```python
from build123d import *

# Parameters (mm, degrees)
BOSS_EXTRUDE1_DEPTH     = 3.175
CUT_EXTRUDE1_DEPTH      = 95.24196383
CUT_EXTRUDE1_DEPTH_BACK = 95.24196383
SKETCH3_W               = 12.7
SKETCH3_H               = 3.175


with BuildPart() as part:
    # Sketch2 → Boss-Extrude1 (new body)
    with BuildSketch(Plane.XY):
        Polygon((13.027299887, 62.53449296), (12.7, 62.861792847), (0, 62.861792847), (0, 0), (70.141728817, 0), (70.141728817, 5.42006403), (67.896664787, 3.175), (58.916408666, 12.155256121), (61.161472696, 14.400320151), (52.181216575, 23.380576272), (49.936152545, 21.135512242), (40.955896424, 30.115768363), (43.200960454, 32.360832393), (34.220704333, 41.341088515), (31.975640303, 39.096024484), (22.995384182, 48.076280605), (25.240448212, 50.321344636), (16.260192091, 59.301600757), (14.015128061, 57.056536726), (10.782235857, 60.28942893), align=None)
    extrude(amount=BOSS_EXTRUDE1_DEPTH)

    # Sketch3 → Cut-Extrude1 (cut, two sides: drawn at the far end of the back side and taken through both)
    with BuildSketch(Plane.XY.offset(3.175).offset(-CUT_EXTRUDE1_DEPTH_BACK)):
        with Locations((44.741728817, 1.5875)):
            Rectangle(SKETCH3_W, SKETCH3_H)
        with Locations((19.341728817, 1.5875)):
            Rectangle(SKETCH3_W, SKETCH3_H)
    extrude(amount=CUT_EXTRUDE1_DEPTH + CUT_EXTRUDE1_DEPTH_BACK, mode=Mode.SUBTRACT)


solid = part.part
```
Work out the finished part from the listing and answer in its coordinate system (mm). A direction names the side the tool comes from. Give positions to 0.01 mm unless a question says otherwise; leave off trailing zeros. Order: outer loops, then holes, each group sorted by start corner. A loop starts at its lowest first (then second) coordinate and runs counter-clockwise, first axis right, second up. Notation, with made-up numbers: M 26,11 L 49,11 A17 cw 49,21 Z; hole C 8.5,-16.5 d6. An arc over 180 degrees is marked long. Return JSON: item names as keys, results as strings.
1) Section D-D, the plane y = 7.5 is taken. Write down the section's boundary in (x, z) (3 decimals).
Resolved:
{"outline": "M 0,0 L 63.572,0 L 63.572,3.175 L 0,3.175 Z"}
2) Section C-C, the plane x = 47 is taken. Write down the section's boundary in (y, z) (3 decimals), plus the area to 3 significant figures.
Resolved:
{"outline": "M 3.175,0 L 24.072,0 L 24.072,3.175 L 3.175,3.175 Z", "area": "66.3 mm^2"}
3) Straight lines are drawn through the part: line 1 along X through (y, z) = (4, 1.3); line 2 along Y through (x, z) = (42, 0.4) (3 decimals); line 3 along X through (y, z) = (58.5, 2.3). For each, find the intervals that lie inside material, in ascending order. Write a range as [from, to].
Resolved:
{"line 1": "[0, 67.07], [68.72, 70.14]", "line 2": "[3.175, 29.072], [31.16, 33.562]", "line 3": "[0, 12.57], [15.46, 17.06]"}
4) Each of these flat-tipped pins is pushed along its axis until it touches: pin 1 (8 mm diameter, centred on x = 48, y = 36, fed in from +Z); pin 2 (1.6 mm diameter, centred on x = 43, z = 1.5, fed in from -Y) (3 decimals). Where does it stop, or does it pass through?
Resolved:
{"pin 1": "through", "pin 2": "y = 3.175"}
5) Section A-A, the plane z = 1.05 is taken. Write down the section's boundary in (x, y) (1 decimal), plus the area to 3 significant figures.
Resolved:
{"outline": "M 0,0 L 13,0 L 13,3.2 L 25.7,3.2 L 25.7,0 L 38.4,0 L 38.4,3.2 L 51.1,3.2 L 51.1,0 L 70.1,0 L 70.1,5.4 L 67.9,3.2 L 58.9,12.2 L 61.2,14.4 L 52.2,23.4 L 49.9,21.1 L 41,30.1 L 43.2,32.4 L 34.2,41.3 L 32,39.1 L 23,48.1 L 25.2,50.3 L 16.3,59.3 L 14,57.1 L 10.8,60.3 L 13,62.5 L 12.7,62.9 L 0,62.9 Z", "area": "2,540 mm^2"}
6) Section B-B, the plane y = 40 is taken. Write down the section's boundary in (x, z) (3 decimals), plus the area to 3 significant figures.
Resolved:
{"outline": "M 0,0 L 31.072,0 L 31.072,3.175 L 0,3.175 Z; M 32.88,0 L 35.562,0 L 35.562,3.175 L 32.88,3.175 Z", "area": "107 mm^2"}
7) A tool of negligible diameter and unlimited length cuts with its end or side. For faces 1 (the flat face through (33.11, 40.23, 1.57)), 2 (the flat face through (45.51, 25.56, 1.57)), 3 (the flat face through (45, 3.175, 2)), 4 (the flat face through (24.1, 49.18, 1.57)), from which of +Z, -Z, +X, -X, +Y, -Y can it reach the whole face along a straight path? Write none if from no direction.
Resolved:
{"face 1": "+Z, -Z, +Y", "face 2": "+Z, -Z", "face 3": "+Z, -Z, -Y", "face 4": "+Z, -Z, +X"}
8) For a pull along X with two mould halves and no side action, classify faces 5 (the flat face through (6, 0, 2)), 6 (the flat face through (69.03, 4.31, 1.57)), 7 (the flat face through (56.73, 18.83, 1.57)) as +X half, -X half, draft (parallel to the pull), parting line (faces both ways), or undercut.
Resolved:
{"face 5": "draft", "face 6": "undercut", "face 7": "+X half"}
